The listing builds one solid part. Answer for the finished solid, in the listing's coordinates (mm). A direction names the side the tool comes from. Give positions to 0.01 mm unless a question says otherwise; leave off trailing zeros. Order: outer loops, then holes, each group sorted by start corner. A loop starts at its lowest first (then second) coordinate and runs counter-clockwise, first axis right, second up. Notation, with made-up numbers: (30.5, 35) - (66.5, 35) arc R17 cw to (66.5, 49) - close; hole circle Ø6 at (-34, 58). An arc over 180 degrees is marked (long way). Write each question's results on one line, items separated by ' | '. Start each with the question number.
1. Which of the six approach directions +Z, -Z, +X, -X, +Y, -Y give full straight-line access (tool end or side, diameter ignored) to faces 1 (the face through (-8, 17, 5)), 2 (the face through (0, -20.5, 5))?
2. Section A-A (x = 19.5) is taken. Give the vertices of the cut face in (y, z).
3. Find the intervals of material crossed by L1, parallel to Y at x = 18, z = 2.25; L2, parallel to Y at x = -5, z = 5; L3, parallel to X at y = 14, z = 7, in increasing order.
4. Section B-B (y = -15) is taken. Give the vertices of the cut face in (x, z).
5. Section C-C (z = 4) is taken. Give the vertices of the cut face in (x, y).
from build123d import *

# Parameters (mm, degrees)
SKETCH1_W           = 50
SKETCH1_H           = 41
BOSS_EXTRUDE1_DEPTH = 10
CUT_EXTRUDE1_DEPTH  = 10


with BuildPart() as part:
    # Sketch1 → Boss-Extrude1 (new body)
    with BuildSketch(Plane.XY):
        Rectangle(SKETCH1_W, SKETCH1_H)
    extrude(amount=BOSS_EXTRUDE1_DEPTH)

    # Sketch2 → Cut-Extrude1 (cut)
    with BuildSketch(Plane(origin=(0, 0, 0), x_dir=(-1, 0, 0), z_dir=(0, 0, -1))):
        with BuildLine():
            Line((9.7, -17), (5.7, -17))
            ThreePointArc((5.7, -17), (3.7, -15), (5.7, -13))
            Line((5.7, -13), (9.7, -13))
            ThreePointArc((9.7, -13), (11.7, -15), (9.7, -17))
        make_face()
        with BuildLine():
            Line((-14.3, -17), (-18.3, -17))
            ThreePointArc((-18.3, -17), (-20.3, -15), (-18.3, -13))
            Line((-18.3, -13), (-14.3, -13))
            ThreePointArc((-14.3, -13), (-12.3, -15), (-14.3, -17))
        make_face()
        with BuildLine():
            Line((5.7, 13), (9.7, 13))
            ThreePointArc((9.7, 13), (11.7, 15), (9.7, 17))
            Line((9.7, 17), (5.7, 17))
            ThreePointArc((5.7, 17), (3.7, 15), (5.7, 13))
        make_face()
        with BuildLine():
            Line((-18.3, 13), (-14.3, 13))
            ThreePointArc((-14.3, 13), (-12.3, 15), (-14.3, 17))
            Line((-14.3, 17), (-18.3, 17))
            ThreePointArc((-18.3, 17), (-20.3, 15), (-18.3, 13))
        make_face()
    extrude(amount=-CUT_EXTRUDE1_DEPTH, mode=Mode.SUBTRACT)


solid = part.part
Reported:
1) face 1: +Z, -Z | face 2: +Z, -Z, +X, -X, -Y
2) outline: (-20.5, 0) - (-16.6, 0) - (-16.6, 10) - (-20.5, 10) - close; (-13.4, 0) - (13.4, 0) - (13.4, 10) - (-13.4, 10) - close; (16.6, 0) - (20.5, 0) - (20.5, 10) - (16.6, 10) - close
3) L1: -20.5 to -17, -13 to 13, 17 to 20.5 | L2: -20.5 to -16.87, -13.13 to 13.13, 16.87 to 20.5 | L3: -25 to -11.43, -3.97 to 12.57, 20.03 to 25
4) outline: (-25, 0) - (-11.7, 0) - (-11.7, 10) - (-25, 10) - close; (-3.7, 0) - (12.3, 0) - (12.3, 10) - (-3.7, 10) - close; (20.3, 0) - (25, 0) - (25, 10) - (20.3, 10) - close
5) outline: (-25, -20.5) - (25, -20.5) - (25, 20.5) - (-25, 20.5) - close; hole (-9.7, -17) - (-5.7, -17) arc R2 ccw to (-5.7, -13) - (-9.7, -13) arc R2 ccw to start; hole (-9.7, 13) - (-5.7, 13) arc R2 ccw to (-5.7, 17) - (-9.7, 17) arc R2 ccw to start; hole (14.3, -17) - (18.3, -17) arc R2 ccw to (18.3, -13) - (14.3, -13) arc R2 ccw to start; hole (14.3, 13) - (18.3, 13) arc R2 ccw to (18.3, 17) - (14.3, 17) arc R2 ccw to start
